```python
from build123d import *

# Parameters (mm, degrees)
F0_W     = 120
F0_H     = 60
F0_R     = 1.65
F0_R_2   = 1.25
F1_DEPTH = 10


with BuildPart() as f1:
    # F0 (on Top) → F1 (new body)
    with BuildSketch(Plane.XY):
        Rectangle(F0_W, F0_H)
        with Locations((-17.5, -17.5)):
            Circle(F0_R, mode=Mode.SUBTRACT)
        with Locations((-50, -13)):
            Circle(F0_R, mode=Mode.SUBTRACT)
        with Locations((50, -13)):
            Circle(F0_R, mode=Mode.SUBTRACT)
        with Locations((0, 22)):
            Circle(F0_R_2, mode=Mode.SUBTRACT)
        with Locations((17.5, 17.5)):
            Circle(F0_R, mode=Mode.SUBTRACT)
    extrude(amount=F1_DEPTH)


solid = f1.part
```
Here's how the part is built. I have some questions about the finished solid (model axes, mm). Coordinates: 2 decimals unless noted, no trailing zeros. Order: outer loops, then holes, each group sorted by start corner. A loop starts at its lowest first (then second) coordinate and runs counter-clockwise, first axis right, second up. Notation, with made-up numbers: M 56.5,8 L 77.5,8 A35 ccw 77.5,43 Z; hole C 16.25,36.5 d4. An arc over 180 degrees is marked long. Answer as a JSON object with one key per item and string values. Group by question number.
(1) I need wall thicknesses on probe 1 along Y at (x, z) = (0, 2.75); probe 2 along Y at (x, z) = (50, 5.25); probe 3 along X at (y, z) = (-16.5, 2.5). Which ranges of each line are inside material? Lowest first, please.
(2) Suppose I cut it at A-A, the plane y = 22. Please give me the cut outline in (x, z).
(3) Suppose I cut it at C-C, the plane y = -13. Please give me the cut outline in (x, z), then the cut area to 3 significant figures.
(4) For pin 1 (2 mm diameter, centred on x = -50, y = -13, fed in from -Z), with a flat end and sliding along its axis, tell me the tip position at first contact or that it passes through.
(5) If we mould it in two halves opening along X, with no side actions, what happens to faces 1 (the face through (60, 0, 5)), 2 (the face through (-1, 0, 10)), 3 (the face through (48.69, -14, 4.93))? For each: released by +X, released by -X, zero draft, split by the parting line, or undercut.
(6) Suppose I cut it at B-B, the plane x = 0. Please give me the cut outline in (y, z), then the cut area to 3 significant figures.
Values found:
{
 "1": {"probe 1": "y = -30 to 20.75, 23.25 to 30", "probe 2": "y = -30 to -14.65, -11.35 to 30", "probe 3": "x = -60 to -18.81, -16.19 to 60"},
 "2": {"outline": "M -60,0 L -1.25,0 L -1.25,10 L -60,10 Z; M 1.25,0 L 60,0 L 60,10 L 1.25,10 Z"},
 "3": {"outline": "M -60,0 L -51.65,0 L -51.65,10 L -60,10 Z; M -48.35,0 L 48.35,0 L 48.35,10 L -48.35,10 Z; M 51.65,0 L 60,0 L 60,10 L 51.65,10 Z", "area": "1,130 mm^2"},
 "4": {"pin 1": "passes through"},
 "5": {"face 1": "released by +X", "face 2": "zero draft", "face 3": "undercut"},
 "6": {"outline": "M -30,0 L 20.75,0 L 20.75,10 L -30,10 Z; M 23.25,0 L 30,0 L 30,10 L 23.25,10 Z", "area": "575 mm^2"}
}
